Geometry: see drawing. Coordinates: mm, zero at the bounding-box minimum. A direction names the side the tool comes from. Give positions to 0.01 mm unless a question says otherwise; leave off trailing zeros. Loops run counter-clockwise (first coordinate to the right, second up) from the corner with the lowest first, then second, coordinate; pieces in that order, holes last. Notation, with made-up numbers: (-28, 78) -> (-4, 78) arc R24 cw to (-4, 103) -> close; hole circle Ø6 at (-26.5, 64). An arc over 180 degrees is marked (long way). Return JSON: item names as keys, results as strings. Group by question number.
(1) Cut plane C-C on y = 6. Return loops of the section in (x, z), then the cut area to 3 significant figures.
(2) Cut plane A-A on z = 2.05. Return loops of the section in (x, y), then the cut area to 3 significant figures.
(3) Access query for the marked faces 1 and 2. Directions: +Z, -Z, +X, -X, +Y, -Y. A direction counts if a zero-diameter tool reaches every point of the face in a straight line with its end or side. Return the directions, or none.
(4) Ray query, line 1 (Y direction, x = 10.5, z = 1.9) (3 decimals); line 2 (X direction, y = 20, z = 3.2); line 3 (Y direction, x = 23, z = 3.9). Return the intervals inside material, ascending. Write a range as from..to.
(5) Cut plane B-B on x = 23. Return loops of the section in (y, z), then the cut area to 4 significant figures.
(6) Pin query (flat end, axial travel): pin 1 (1 mm diameter, centred on y = 8, z = 3.5, fed in from +X); pin 2 (3 mm diameter, centred on x = 24, z = 1.5, fed in from +Y) (3 decimals); pin 3 (1.5 mm diameter, centred on x = 43.5, z = 2, fed in from -Y). Return the tip coordinate at first contact, or that it passes through.
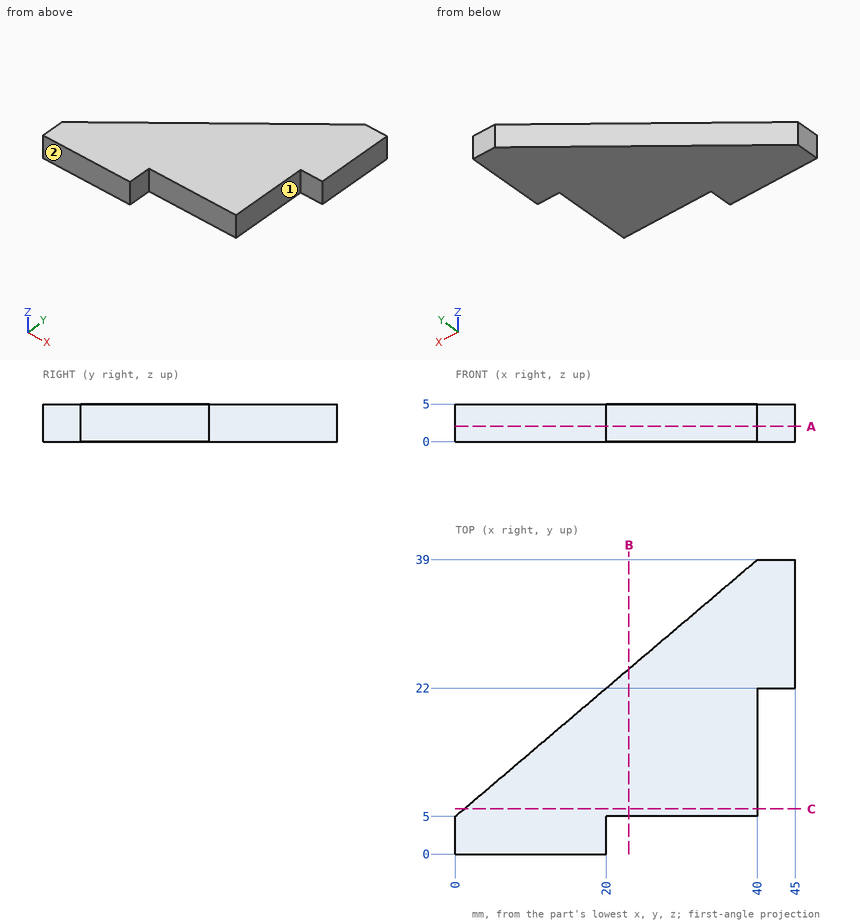
Answers:
{
 "1": {"outline": "(1.18, 0) -> (40, 0) -> (40, 5) -> (1.18, 5) -> close", "area": "194 mm²"},
 "2": {"outline": "(0, 0) -> (20, 0) -> (20, 5) -> (40, 5) -> (40, 22) -> (45, 22) -> (45, 39) -> (40, 39) -> (0, 5) -> close", "area": "865 mm²"},
 "3": {"face 1": "+Z, -Z, +X, -Y", "face 2": "+Z, -Z, +X, -X, -Y"},
 "4": {"line 1": "0..13.925", "line 2": "17.65..40", "line 3": "5..24.55"},
 "5": {"outline": "(5, 0) -> (24.55, 0) -> (24.55, 5) -> (5, 5) -> close", "area": "97.75 mm²"},
 "6": {"pin 1": "x = 40", "pin 2": "y = 26.675", "pin 3": "y = 22"}
}
